from build123d import *

# Parameters (mm, degrees)
BOSS_EXTRUDE1_DEPTH   = 30
SKETCH2_R             = 9.5
SKETCH2_R_2           = 1.5
BOSS_EXTRUDE2_DEPTH   = 7
BOSS_EXTRUDE2_2_DEPTH = 7
BOSS_EXTRUDE3_START   = -2
SKETCH3_3_R           = 2
BOSS_EXTRUDE3_DEPTH   = 2
SKETCH2_5_R           = 6
CUT_EXTRUDE2_DEPTH    = 3
SKETCH3_6_R           = 3.5
BOSS_EXTRUDE15_DEPTH  = 20
SKETCH3_10_R          = 3.5
SKETCH3_10_R_2        = 2
BOSS_EXTRUDE16_DEPTH  = 15
CUT_EXTRUDE3_START    = -2
SKETCH3_11_R          = 3.5
CUT_EXTRUDE3_DEPTH    = 3
LPATTERN3_COUNT       = 3
LPATTERN3_PITCH       = 110
LPATTERN3_COL_COUNT   = 3
LPATTERN3_COL_PITCH   = 110


with BuildPart() as part:
    # Sketch3 → Boss-Extrude1 (new body)
    with BuildSketch(Plane(origin=(0, 0, 0), x_dir=(1, 0, 0), z_dir=(0, 1, 0))):
        with BuildLine():
            Line((220, 31), (-220, 31))
            ThreePointArc((-220, 31), (-251, 0), (-220, -31))
            Line((-220, -31), (220, -31))
            ThreePointArc((220, -31), (251, 0), (220, 31))
        make_face()
        with BuildLine():
            Line((220, -29), (-220, -29))
            ThreePointArc((-220, -29), (-249, 0), (-220, 29))
            Line((-220, 29), (220, 29))
            ThreePointArc((220, 29), (249, 0), (220, -29))
        make_face(mode=Mode.SUBTRACT)
    extrude(amount=BOSS_EXTRUDE1_DEPTH)



with BuildPart() as body_2:
    # Sketch2 → Boss-Extrude2 (new body)
    with BuildSketch(Plane(origin=(0, 0, 0), x_dir=(1, 0, 0), z_dir=(0, 1, 0))):
        with BuildLine():
            ThreePointArc((230.710286287, 4.188050578), (230.58255933, 5.71944158), (231.313708499, 7.071067812))
            ThreePointArc((231.313708499, 7.071067812), (231.313708499, 11.313708499), (227.071067812, 11.313708499))
            ThreePointArc((227.071067812, 11.313708499), (225.71944158, 10.58255933), (224.188050578, 10.710286287))
            ThreePointArc((224.188050578, 10.710286287), (220, 11.5), (215.811949422, 10.710286287))
            ThreePointArc((215.811949422, 10.710286287), (214.28055842, 10.58255933), (212.928932188, 11.313708499))
            ThreePointArc((212.928932188, 11.313708499), (208.686291501, 11.313708499), (208.686291501, 7.071067812))
            ThreePointArc((208.686291501, 7.071067812), (209.41744067, 5.71944158), (209.289713713, 4.188050578))
            ThreePointArc((209.289713713, 4.188050578), (208.5, 0), (209.289713713, -4.188050578))
            ThreePointArc((209.289713713, -4.188050578), (209.41744067, -5.71944158), (208.686291501, -7.071067812))
            ThreePointArc((208.686291501, -7.071067812), (208.686291501, -11.313708499), (212.928932188, -11.313708499))
            ThreePointArc((212.928932188, -11.313708499), (214.28055842, -10.58255933), (215.811949422, -10.710286287))
            ThreePointArc((215.811949422, -10.710286287), (220, -11.5), (224.188050578, -10.710286287))
            ThreePointArc((224.188050578, -10.710286287), (225.71944158, -10.58255933), (227.071067812, -11.313708499))
            ThreePointArc((227.071067812, -11.313708499), (231.313708499, -11.313708499), (231.313708499, -7.071067812))
            ThreePointArc((231.313708499, -7.071067812), (230.58255933, -5.71944158), (230.710286287, -4.188050578))
            ThreePointArc((230.710286287, -4.188050578), (231.5, 0), (230.710286287, 4.188050578))
        make_face()
        with Locations(Location((220, 0, 0), (0, 0, 270))):
            Circle(SKETCH2_R, mode=Mode.SUBTRACT)
        with Locations(Location((229.192388155, 9.192388155, 0), (0, 0, 270))):
            Circle(SKETCH2_R_2, mode=Mode.SUBTRACT)
        with Locations(Location((229.192388155, -9.192388155, 0), (0, 0, 270))):
            Circle(SKETCH2_R_2, mode=Mode.SUBTRACT)
        with Locations(Location((210.807611845, 9.192388155, 0), (0, 0, 270))):
            Circle(SKETCH2_R_2, mode=Mode.SUBTRACT)
        with Locations(Location((210.807611845, -9.192388155, 0), (0, 0, 270))):
            Circle(SKETCH2_R_2, mode=Mode.SUBTRACT)
    extrude(amount=BOSS_EXTRUDE2_DEPTH)


with BuildPart() as body_3:
    # Sketch2 → Boss-Extrude2 2 (new body)
    with BuildSketch(Plane(origin=(0, 0, 0), x_dir=(1, 0, 0), z_dir=(0, 1, 0))):
        with BuildLine():
            ThreePointArc((-208.686291501, 7.071067812), (-208.686291501, 11.313708499), (-212.928932188, 11.313708499))
            ThreePointArc((-212.928932188, 11.313708499), (-214.28055842, 10.58255933), (-215.811949422, 10.710286287))
            ThreePointArc((-215.811949422, 10.710286287), (-220, 11.5), (-224.188050578, 10.710286287))
            ThreePointArc((-224.188050578, 10.710286287), (-225.71944158, 10.58255933), (-227.071067812, 11.313708499))
            ThreePointArc((-227.071067812, 11.313708499), (-231.313708499, 11.313708499), (-231.313708499, 7.071067812))
            ThreePointArc((-231.313708499, 7.071067812), (-230.58255933, 5.71944158), (-230.710286287, 4.188050578))
            ThreePointArc((-230.710286287, 4.188050578), (-231.5, 0), (-230.710286287, -4.188050578))
            ThreePointArc((-230.710286287, -4.188050578), (-230.58255933, -5.71944158), (-231.313708499, -7.071067812))
            ThreePointArc((-231.313708499, -7.071067812), (-231.313708499, -11.313708499), (-227.071067812, -11.313708499))
            ThreePointArc((-227.071067812, -11.313708499), (-225.71944158, -10.58255933), (-224.188050578, -10.710286287))
            ThreePointArc((-224.188050578, -10.710286287), (-220, -11.5), (-215.811949422, -10.710286287))
            ThreePointArc((-215.811949422, -10.710286287), (-214.28055842, -10.58255933), (-212.928932188, -11.313708499))
            ThreePointArc((-212.928932188, -11.313708499), (-208.686291501, -11.313708499), (-208.686291501, -7.071067812))
            ThreePointArc((-208.686291501, -7.071067812), (-209.41744067, -5.71944158), (-209.289713713, -4.188050578))
            ThreePointArc((-209.289713713, -4.188050578), (-208.5, 0), (-209.289713713, 4.188050578))
            ThreePointArc((-209.289713713, 4.188050578), (-209.41744067, 5.71944158), (-208.686291501, 7.071067812))
        make_face()
        with Locations(Location((-210.807611845, 9.192388155, 0), (0, 0, 270))):
            Circle(SKETCH2_R_2, mode=Mode.SUBTRACT)
        with Locations(Location((-220, 0, 0), (0, 0, 270))):
            Circle(SKETCH2_R, mode=Mode.SUBTRACT)
        with Locations(Location((-229.192388155, 9.192388155, 0), (0, 0, 270))):
            Circle(SKETCH2_R_2, mode=Mode.SUBTRACT)
        with Locations(Location((-210.807611845, -9.192388155, 0), (0, 0, 270))):
            Circle(SKETCH2_R_2, mode=Mode.SUBTRACT)
        with Locations(Location((-229.192388155, -9.192388155, 0), (0, 0, 270))):
            Circle(SKETCH2_R_2, mode=Mode.SUBTRACT)
    extrude(amount=BOSS_EXTRUDE2_2_DEPTH)


with BuildPart() as part_1:
    add(part.part)

    add(body_2.part)  # Boss-Extrude3 merges body 2

    add(body_3.part)  # Boss-Extrude3 merges body 3
    # Sketch3<3> → Boss-Extrude3 (add)
    with BuildSketch(Plane(origin=(0, 0, 0), x_dir=(1, 0, 0), z_dir=(0, 1, 0)).offset(BOSS_EXTRUDE3_START)):
        with BuildLine():
            Line((220, 31), (-220, 31))
            ThreePointArc((-220, 31), (-251, 0), (-220, -31))
            Line((-220, -31), (220, -31))
            ThreePointArc((220, -31), (251, 0), (220, 31))
        make_face()
        with Locations(Location((0, 25.25, 0), (0, 0, 270))):
            Circle(SKETCH3_3_R, mode=Mode.SUBTRACT)
        with Locations(Location((0, -25.25, 0), (0, 0, 270))):
            Circle(SKETCH3_3_R, mode=Mode.SUBTRACT)
    boss_extrude3 = extrude(amount=BOSS_EXTRUDE3_DEPTH)

    # Mirror4: Boss-Extrude3 across plane
    add(boss_extrude3.mirror(Plane(origin=(0, 0, 0), x_dir=(0, 0, 1), z_dir=(1, 0, 0))))

    # Sketch2<5> → Cut-Extrude2 (cut)
    with BuildSketch(Plane(origin=(0, 0, 0), x_dir=(1, 0, 0), z_dir=(0, 1, 0))):
        with Locations(Location((220, 0, 0), (0, 0, 270))):
            Circle(SKETCH2_5_R)
        with Locations(Location((-220, 0, 0), (0, 0, 270))):
            Circle(SKETCH2_5_R)
    extrude(amount=-CUT_EXTRUDE2_DEPTH, mode=Mode.SUBTRACT)

    # Sketch3<6> → Boss-Extrude15 (add)
    # profile 1 of 2: a face of its own
    with BuildSketch(Plane(origin=(0, 0, 0), x_dir=(1, 0, 0), z_dir=(0, 1, 0))):
        with BuildLine():
            ThreePointArc((-3.307189139, 29), (0, 20.25), (3.307189139, 29))
            Line((3.307189139, 29), (-3.307189139, 29))
        make_face()
        with Locations(Location((0, 25.25, 0), (0, 0, 270))):
            Circle(SKETCH3_6_R, mode=Mode.SUBTRACT)
    # profile 2 of 2: a face of its own
    with BuildSketch(Plane(origin=(0, 0, 0), x_dir=(1, 0, 0), z_dir=(0, 1, 0))):
        with BuildLine():
            Line((-3.307189139, -29), (3.307189139, -29))
            ThreePointArc((3.307189139, -29), (0, -20.25), (-3.307189139, -29))
        make_face()
        with Locations(Location((0, -25.25, 0), (0, 0, 270))):
            Circle(SKETCH3_6_R, mode=Mode.SUBTRACT)
    boss_extrude15 = extrude(amount=BOSS_EXTRUDE15_DEPTH)

    # Sketch3<10> → Boss-Extrude16 (add)
    # profile 1 of 2: a face of its own
    with BuildSketch(Plane(origin=(0, 0, 0), x_dir=(1, 0, 0), z_dir=(0, 1, 0))):
        with Locations(Location((0, -25.25, 0), (0, 0, 270))):
            Circle(SKETCH3_10_R)
        with Locations(Location((0, -25.25, 0), (0, 0, 270))):
            Circle(SKETCH3_10_R_2, mode=Mode.SUBTRACT)
    # profile 2 of 2: a face of its own
    with BuildSketch(Plane(origin=(0, 0, 0), x_dir=(1, 0, 0), z_dir=(0, 1, 0))):
        with Locations(Location((0, 25.25, 0), (0, 0, 270))):
            Circle(SKETCH3_10_R)
        with Locations(Location((0, 25.25, 0), (0, 0, 270))):
            Circle(SKETCH3_10_R_2, mode=Mode.SUBTRACT)
    boss_extrude16 = extrude(amount=BOSS_EXTRUDE16_DEPTH)

    # Sketch3<11> → Cut-Extrude3 (cut)
    with BuildSketch(Plane(origin=(0, 0, 0), x_dir=(1, 0, 0), z_dir=(0, 1, 0)).offset(CUT_EXTRUDE3_START)):
        with Locations(Location((0, 25.25, 0), (0, 0, 270))):
            Circle(SKETCH3_11_R)
        with Locations(Location((0, -25.25, 0), (0, 0, 270))):
            Circle(SKETCH3_11_R)
    cut_extrude3 = extrude(amount=CUT_EXTRUDE3_DEPTH, mode=Mode.SUBTRACT)

    # LPattern3: Boss-Extrude15, Boss-Extrude16, Cut-Extrude3 ×3
    with Locations(*[(i * LPATTERN3_PITCH, 0, 0) for i in range(1, LPATTERN3_COUNT)]):
        add(boss_extrude15)
        add(boss_extrude16)
        add(cut_extrude3, mode=Mode.SUBTRACT)

    # LPattern3 col: Boss-Extrude15, Boss-Extrude16, Cut-Extrude3 ×3
    with Locations(*[(-i * LPATTERN3_COL_PITCH, 0, 0) for i in range(1, LPATTERN3_COL_COUNT)]):
        add(boss_extrude15)
        add(boss_extrude16)
        add(cut_extrude3, mode=Mode.SUBTRACT)


solid = part_1.part
Source: CAD feature listing. Evaluate the final solid. Frame: model axes, mm. A direction names the side the tool comes from. Round coordinates to 2 decimals unless told otherwise and drop trailing zeros. Loops run counter-clockwise (first coordinate to the right, second up) from the corner with the lowest first, then second, coordinate; pieces in that order, holes last.
Q1. Section B-B, the plane z = 0. State how many separate pieces and enclosed holes the cut face has, plus the area to 3 significant figures.
Q2. Section A-A, the plane y = 25.5. Return loops of the section in (x, z), plus the area to 3 significant figures.
Q3. Access query for faces 1 (the face through (3, 21, 29)), 2 (the face through (3, 14, -31)). Directions: +Z, -Z, +X, -X, +Y, -Y. A direction counts if a zero-diameter tool reaches every point of the face in a straight line with its end or side. Return the directions, or none.
Q4. Mould query, pull axis X, two halves, no side actions, for faces 3 (the face through (-250.993, 13.776, -0.682)), 4 (the face through (250.993, 13.776, 0.682)), 5 (the face through (-219.67, 9.86, 20.26)). Classes: pulls with the +X half, pulls with the -X half, needs draft (parallel to the pull), parting line crosses it, or undercut.
Q5. Section C-C, the plane x = -173. Return loops of the section in (y, z), plus the area to 3 significant figures.
Q6. First-contact query: P1, Ø4.5, axis at x = -109.5, z = -26.5, coming from the +Y side; P2, Ø2, axis at x = 0.5, z = -26.5, coming from the -Y side; P3, Ø5.5, axis at x = -110, z = -25.25, coming from the +Y side. Flat tips, straight axial feed; report the tip coordinate or a pass-through.
Q7. Ray query, line 1 (Z direction, x = -220, y = 17.2); line 2 (X direction, y = 4, z = -0.5); line 3 (X direction, y = 28, z = -0.5). Return the intervals inside material, ascending.
Solutions:
1. separate pieces: 3
1. enclosed holes: 0
1. area: 1,130 mm2
2. outline: (-220, -31) - (220, -31) arc R31 ccw to (220, 31) - (-220, 31) arc R31 ccw to start; hole (-220, -29) - (220, -29) arc R29 ccw to (220, 29) - (-220, 29) arc R29 ccw to start
2. area: 2,140 mm2
3. face 1: +Y
3. face 2: -Z, +X, -X, +Y, -Y
4. face 3: pulls with the -X half
4. face 4: pulls with the +X half
4. face 5: undercut
5. outline: (-2, -31) - (30, -31) - (30, -29) - (0, -29) - (0, 29) - (30, 29) - (30, 31) - (-2, 31) - close
5. area: 244 mm2
6. P1: stops at y = 20
6. P2: stops at y = 1
6. P3: stops at y = 15
7. line 1: z = -31 to -28.75, -21.75 to -20.25, 20.25 to 21.75, 28.75 to 31
7. line 2: x = -251 to -249, -231.49 to -229.49, -210.51 to -208.51, 208.51 to 210.51, 229.49 to 231.49, 249 to 251
7. line 3: x = -251 to -249, 249 to 251
